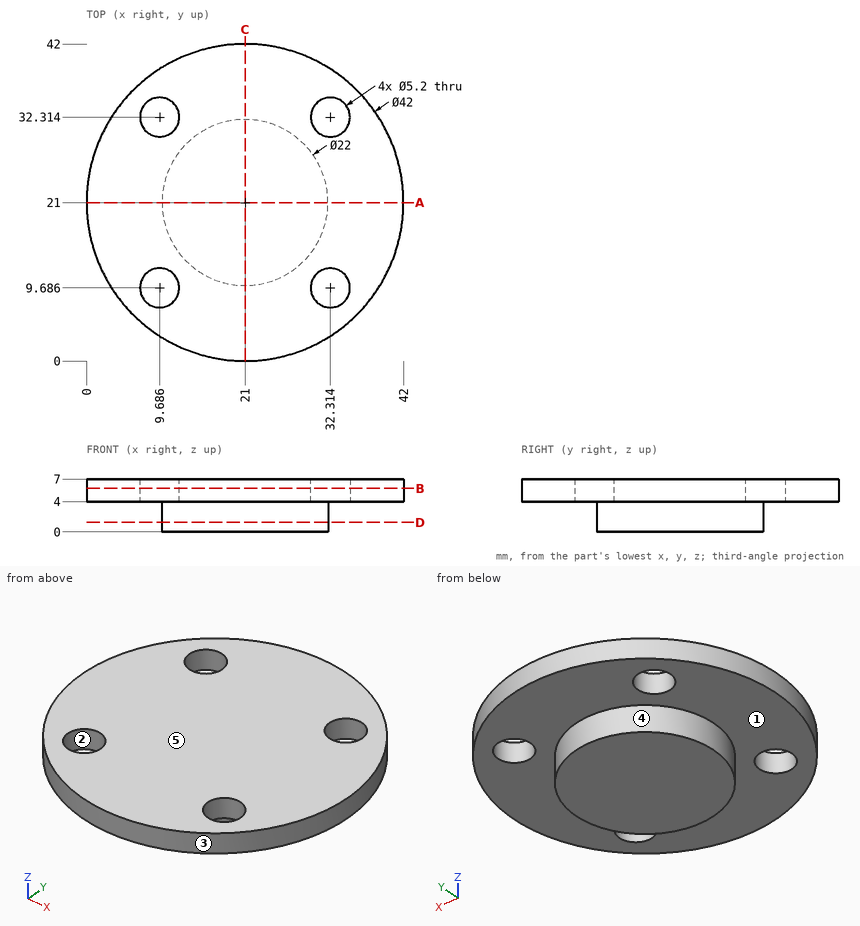
Geometry check sheet. Reference: drawing and pictorial views, mm from the part's lowest x, y, z. A direction names the side the tool comes from. Round coordinates to 2 decimals unless told otherwise and drop trailing zeros. Loops run counter-clockwise (first coordinate to the right, second up) from the corner with the lowest first, then second, coordinate; pieces in that order, holes last. Notation, with made-up numbers: (1.5, 86) -> (42.5, 86) arc R12 ccw to (42.5, 99) -> close; hole circle Ø4 at (40, 67.25). An arc over 180 degrees is marked (long way). Use a Markdown table: item, result.
(1) Scan lines: probe 1 along X at (y, z) = (10, 6) (1 decimal); probe 2 along Y at (x, z) = (33, 4.75) (1 decimal); probe 3 along Z at (x, y) = (33.5, 12.5). Record each from-to range of solid material in increasing order.
Calculated:
| item | result |
|---|---|
| probe 1 | 3.1 to 7.1, 12.3 to 29.7, 34.9 to 38.9 |
| probe 2 | 3.8 to 7.2, 12.2 to 29.8, 34.8 to 38.2 |
| probe 3 | 4 to 7 |
(2) Set-up check for the marked faces 4 and 5: record each of +Z, -Z, +X, -X, +Y, -Y from which the full face is reachable in a straight line by a thin tool's end or side.
Calculated:
| item | result |
|---|---|
| face 4 | -Z |
| face 5 | +Z, +X, -X, +Y, -Y |
(3) Sectioned sample at B-B (z = 5.75). Enter the section's corners in (x, y), then the cut area to 3 significant figures.
Calculated:
| item | result |
|---|---|
| outline | circle Ø42 at (21, 21); hole circle Ø5.2 at (9.69, 9.69); hole circle Ø5.2 at (9.69, 32.31); hole circle Ø5.2 at (32.31, 9.69); hole circle Ø5.2 at (32.31, 32.31) |
| area | 1,300 mm² |
(4) Sectioned sample at A-A (y = 21). Enter the section's corners in (x, z).
Calculated:
| item | result |
|---|---|
| outline | (0, 4) -> (10, 4) -> (10, 0) -> (32, 0) -> (32, 4) -> (42, 4) -> (42, 7) -> (0, 7) -> close |
(5) Sectioned sample at D-D (z = 1.25). Enter the section's corners in (x, y).
Calculated:
| item | result |
|---|---|
| outline | circle Ø22 at (21, 21) |
(6) Go/stop test with flat-tipped pins: P1, Ø4, axis at y = 5, z = 3.5, coming from the -X side (1 decimal); P2, Ø4, axis at y = 8.5, z = 2.5, coming from the -X side. Record where each tip stops, or that it passes through.
Calculated:
| item | result |
|---|---|
| P1 | x = 5.4 |
| P2 | x = 3.22 |
(7) Mould release check, pull along Y, two halves, no side actions. Record for the marked faces 1, 2 and 3: released by +Y, released by -Y, zero draft, split by the parting line, or undercut.
Calculated:
| item | result |
|---|---|
| face 1 | zero draft |
| face 2 | undercut |
| face 3 | split by the parting line |
